```python
from build123d import *

# Parameters (mm, degrees)
SKETCH1_W           = 95
SKETCH1_H           = 65
BOSS_EXTRUDE1_DEPTH = 5
SKETCH3_W           = 90
SKETCH3_H           = 60
CUT_EXTRUDE1_DEPTH  = 2.5
SKETCH5_W           = 15
SKETCH5_H           = 5
BOSS_EXTRUDE2_DEPTH = 2.1
SKETCH14_W          = 13
SKETCH14_H          = 2
CUT_EXTRUDE3_DEPTH  = 2.5
CUT_EXTRUDE5_REACH  = 117.217
SKETCH17_W          = 24
SKETCH17_H          = 2.5
SKETCH18_R          = 0.65
CUT_EXTRUDE6_DEPTH  = 2.5
SKETCH19_W          = 7.5
SKETCH19_H          = 5
BOSS_EXTRUDE3_DEPTH = 7.5
SKETCH20_W          = 7.5
SKETCH20_H          = 5
BOSS_EXTRUDE4_DEPTH = 7.5
SKETCH21_R          = 1.65
CUT_EXTRUDE7_DEPTH  = 122.475306133


with BuildPart() as part:
    # Sketch1 → Boss-Extrude1 (new body)
    with BuildSketch(Plane(origin=(0, 0, 0), x_dir=(1, 0, 0), z_dir=(0, 1, 0))):
        with Locations((47.5, 32.5)):
            Rectangle(SKETCH1_W, SKETCH1_H)
    extrude(amount=-BOSS_EXTRUDE1_DEPTH)

    # Sketch3 → Cut-Extrude1 (cut)
    with BuildSketch(Plane(origin=(0, 0, 0), x_dir=(1, 0, 0), z_dir=(0, 1, 0))):
        with Locations((47.5, 32.5)):
            Rectangle(SKETCH3_W, SKETCH3_H)
    extrude(amount=-CUT_EXTRUDE1_DEPTH, mode=Mode.SUBTRACT)

    # Sketch5 → Boss-Extrude2 (add)
    with BuildSketch(Plane(origin=(0, -2.5, 0), x_dir=(1, 0, 0), z_dir=(0, 1, 0))):
        with Locations((10, 60)):
            Rectangle(SKETCH5_W, SKETCH5_H)
        with Locations((10, 5)):
            Rectangle(SKETCH5_W, SKETCH5_H)
        with Locations((85, 60)):
            Rectangle(SKETCH5_W, SKETCH5_H)
        with Locations((85, 5)):
            Rectangle(SKETCH5_W, SKETCH5_H)
    extrude(amount=BOSS_EXTRUDE2_DEPTH)

    # Sketch14 → Cut-Extrude3 (cut)
    with BuildSketch(Plane.XY):
        with Locations((61, -1)):
            Rectangle(SKETCH14_W, SKETCH14_H)
    extrude(amount=-CUT_EXTRUDE3_DEPTH, mode=Mode.SUBTRACT)

    # Sketch17 → Cut-Extrude5 (cut, up to next)
    with BuildSketch(Plane(origin=(95, 0, 0), x_dir=(0, 0, -1), z_dir=(1, 0, 0)), mode=Mode.PRIVATE) as cut_extrude5_sk1:
        with Locations((22, -1.25)):
            Rectangle(SKETCH17_W, SKETCH17_H)
    cut_extrude5_tool1 = extrude(cut_extrude5_sk1.sketch, amount=-CUT_EXTRUDE5_REACH, mode=Mode.PRIVATE) & part.part
    add(cut_extrude5_tool1.solids().sort_by_distance((95, -1.25, -22))[0], mode=Mode.SUBTRACT)

    # Sketch18 → Cut-Extrude6 (cut)
    with BuildSketch(Plane(origin=(0, 0, 0), x_dir=(1, 0, 0), z_dir=(0, 1, 0))):
        with Locations(Location((91.75, 63.75, 0), (0, 0, 270))):
            Circle(SKETCH18_R)
        with Locations(Location((86.75, 63.75, 0), (0, 0, 270))):
            Circle(SKETCH18_R)
        with Locations(Location((91.75, 1.25, 0), (0, 0, 90))):
            Circle(SKETCH18_R)
        with Locations(Location((26, 63.75, 0), (0, 0, 90))):
            Circle(SKETCH18_R)
        with Locations(Location((31, 63.75, 0), (0, 0, 90))):
            Circle(SKETCH18_R)
        with Locations(Location((26, 1.25, 0), (0, 0, 270))):
            Circle(SKETCH18_R)
        with Locations(Location((31, 1.25, 0), (0, 0, 270))):
            Circle(SKETCH18_R)
    extrude(amount=-CUT_EXTRUDE6_DEPTH, mode=Mode.SUBTRACT)

    # Sketch19 → Boss-Extrude3 (add)
    with BuildSketch(Plane.ZY):
        with Locations((-61.25, -2.5)):
            Rectangle(SKETCH19_W, SKETCH19_H)
        with Locations((-3.75, -2.5)):
            Rectangle(SKETCH19_W, SKETCH19_H)
    extrude(amount=BOSS_EXTRUDE3_DEPTH)

    # Sketch20 → Boss-Extrude4 (add)
    with BuildSketch(Plane(origin=(95, 0, 0), x_dir=(0, 0, -1), z_dir=(1, 0, 0))):
        with Locations((3.75, -2.5)):
            Rectangle(SKETCH20_W, SKETCH20_H)
        with Locations((61.25, -2.5)):
            Rectangle(SKETCH20_W, SKETCH20_H)
    extrude(amount=BOSS_EXTRUDE4_DEPTH)

    # Sketch21 → Cut-Extrude7 (cut, through all)
    with BuildSketch(Plane(origin=(0, 0, 0), x_dir=(1, 0, 0), z_dir=(0, 1, 0))):
        with Locations(Location((-3.75, 61.25, 0), (0, 0, 270))):
            Circle(SKETCH21_R)
        with Locations(Location((98.75, 61.25, 0), (0, 0, 90))):
            Circle(SKETCH21_R)
        with Locations(Location((98.75, 3.75, 0), (0, 0, 270))):
            Circle(SKETCH21_R)
        with Locations(Location((-3.75, 3.75, 0), (0, 0, 90))):
            Circle(SKETCH21_R)
    extrude(amount=-CUT_EXTRUDE7_DEPTH, mode=Mode.SUBTRACT)


solid = part.part
```
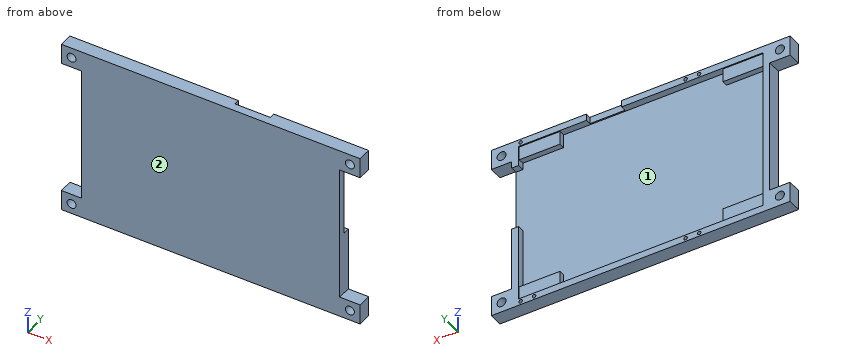
The model under review builds one solid part; all positions refer to its coordinate system, in mm. Face numbers are marked on the shaded views. Give positions to 0.01 mm unless a question says otherwise; leave off trailing zeros. Write each loop counter-clockwise with the first axis right and the second up, starting at its lowest first coordinate (ties: lowest second). Pieces come first, ordered by that corner, then holes. Notation, with made-up numbers: M 84.25,-31 L 139.25,-31 A15 ccw 139.25,-21 Z; hole C -12,-13 d10. An arc over 180 degrees is marked long. Write each question's results on one line, items separated by ' | '. Start each with the question number.
1. Mouldability with a two-part tool opening along Z and no side actions: class the marked faces 1 and 2 as released by +Z, released by -Z, zero draft, split by the parting line, or undercut.
2. Insertion check: pin 1 Ø5 at (x, z) = (3.5, -10) entering from +Y; pin 2 Ø4 at (x, z) = (49.5, -23) entering from +Y; pin 3 Ø0.8 at (x, z) = (59, -1.5) entering from +Y; pin 4 Ø4 at (x, z) = (85, -5.5) entering from +Y. Each pin has a flat end and moves straight along its axis. Give the tip position at first contact, or say it passes through.
3. We need section D-D (z = -51). Write out the cut boundary in (x, y), and give its area (3 significant figures).
4. We need section A-A (x = -3.75). Write out the cut boundary in (y, z), and give its area (3 significant figures).
5. For probe 1 along X at (y, z) = (-1.55, -1.25); probe 2 along X at (y, z) = (-1.05, -63.75); probe 3 along Z at (x, y) = (98.75, -2.1), list the stretches that pass through material, from the lowest coordinate up. Write a range as [from, to].
6. We need section B-B (z = -61.25). Write out the cut boundary in (x, y).
7. We need section C-C (x = 37.5). Write out the cut boundary in (y, z).
Results found:
1) face 1: undercut | face 2: zero draft
2) pin 1: stops at y = 0 | pin 2: stops at y = -2.5 | pin 3: stops at y = -2 | pin 4: stops at y = -0.4
3) outline: M 0,-5 L 95,-5 L 95,0 L 92.5,0 L 92.5,-2.5 L 2.5,-2.5 L 2.5,0 L 0,0 Z | area: 250 mm^2
4) outline: M -5,-65 L 0,-65 L 0,-62.9 L -5,-62.9 Z; M -5,-59.6 L 0,-59.6 L 0,-57.5 L -5,-57.5 Z; M -5,-7.5 L 0,-7.5 L 0,-5.4 L -5,-5.4 Z; M -5,-2.1 L 0,-2.1 L 0,0 L -5,0 Z | area: 42.0 mm^2
5) probe 1: x = [-7.5, 25.35], [26.65, 30.35], [31.65, 54.5], [67.5, 91.1], [92.4, 102.5] | probe 2: x = [-7.5, 25.35], [26.65, 30.35], [31.65, 86.1], [87.4, 91.1], [92.4, 102.5] | probe 3: z = [-65, -62.9], [-59.6, -57.5], [-7.5, -5.4], [-2.1, 0]
6) outline: M -7.5,-5 L -5.4,-5 L -5.4,0 L -7.5,0 Z; M -2.1,-5 L 97.1,-5 L 97.1,0 L 92.5,0 L 92.5,-0.4 L 77.5,-0.4 L 77.5,-2.5 L 17.5,-2.5 L 17.5,-0.4 L 2.5,-0.4 L 2.5,0 L -2.1,0 Z; M 100.4,-5 L 102.5,-5 L 102.5,0 L 100.4,0 Z
7) outline: M -5,-65 L 0,-65 L 0,-62.5 L -2.5,-62.5 L -2.5,-2.5 L 0,-2.5 L 0,0 L -5,0 Z
